```python
from build123d import *

# Parameters (mm, degrees)
F1_DEPTH = 6.3
F3_DEPTH = 4
F4_R     = 2.35
F4_R_2   = 1
F5_DEPTH = 3
F7_DEPTH = 2.5


with BuildPart() as f1:
    # F0 (on Top) → F1 (new body, symmetric)
    with BuildSketch(Plane.XY):
        Polygon((7.7, 11.4), (-8, 11.4), (-8, -11.4), (7.7, -11.4), (7.7, -16.25), (10.2, -16.25), (10.2, -11.4), (15, -11.4), (15, 11.4), (10.2, 11.4), (10.2, 16.25), (7.7, 16.25), align=None)
    extrude(amount=F1_DEPTH, both=True)

    # F2 (on face) → F3 (join)
    with BuildSketch(Plane.YZ.offset(15)):
        with BuildLine():
            ThreePointArc((5.1, 6.3), (1.0729415714, 4.844873622), (-1.0938378269, 1.1516826707))
            ThreePointArc((-1.0938378269, 1.1516826707), (-1.2, 0), (-1.0938378269, -1.1516826707))
            ThreePointArc((-1.0938378269, -1.1516826707), (1.072941559, -4.8448736116), (5.0999999676, -6.3))
            ThreePointArc((5.0999999676, -6.3), (9.55477271, -4.4547727329), (11.4, 0))
            ThreePointArc((11.4, 0), (9.5547727215, 4.4547727215), (5.1, 6.3))
        make_face()
        with BuildLine():
            ThreePointArc((-1.0938378269, -1.1516826707), (-1.2, 0), (-1.0938378269, 1.1516826707))
            ThreePointArc((-1.0938378269, 1.1516826707), (-2.8, 0), (-1.0938378269, -1.1516826707))
        make_face()
    extrude(amount=F3_DEPTH)

    # F4 (on face) → F5 (join)
    with BuildSketch(Plane.YZ.offset(19)):
        with Locations((5.1, 0)):
            Circle(F4_R)
        with Locations((5.1, 0)):
            Circle(F4_R_2, mode=Mode.SUBTRACT)
    extrude(amount=F5_DEPTH)

    # F6 (on face) → F7 (cut, through all)
    with BuildSketch(Plane.YZ.offset(10.2)):
        with BuildLine():
            ThreePointArc((14.6160254038, -0.5), (14.7159258263, -0.2588190451), (14.75, 0))
            ThreePointArc((14.75, 0), (14.7159258263, 0.2588190451), (14.6160254038, 0.5))
            ThreePointArc((14.6160254038, 0.5), (12.75, 0), (14.6160254038, -0.5))
        make_face()
        with BuildLine():
            ThreePointArc((14.6160254038, 0.5), (14.7159258263, 0.2588190451), (14.75, 0))
            ThreePointArc((14.75, 0), (14.7159258263, -0.2588190451), (14.6160254038, -0.5))
            Line((14.6160254038, -0.5), (16.25, -0.5))
            Line((16.25, -0.5), (16.25, 0.5))
            Line((16.25, 0.5), (14.6160254038, 0.5))
        make_face()
        with BuildLine():
            ThreePointArc((-14.6160254038, -0.5), (-13.4911809549, -0.9659258263), (-12.75, 0))
            ThreePointArc((-12.75, 0), (-13.4911809549, 0.9659258263), (-14.6160254038, 0.5))
            ThreePointArc((-14.6160254038, 0.5), (-14.75, 0), (-14.6160254038, -0.5))
        make_face()
        with BuildLine():
            ThreePointArc((-14.6160254038, -0.5), (-14.75, 0), (-14.6160254038, 0.5))
            Line((-14.6160254038, 0.5), (-16.25, 0.5))
            Line((-16.25, 0.5), (-16.25, -0.5))
            Line((-16.25, -0.5), (-14.6160254038, -0.5))
        make_face()
    extrude(amount=-F7_DEPTH, mode=Mode.SUBTRACT)


solid = f1.part
```
Can you work these out from the model? Positions are in its coordinate system, mm. A direction names the side the tool comes from. Round coordinates to 2 decimals unless told otherwise and drop trailing zeros. Order: outer loops, then holes, each group sorted by start corner. A loop starts at its lowest first (then second) coordinate and runs counter-clockwise, first axis right, second up. Notation, with made-up numbers: (-40, 49) -> (16, 49) arc R20 ccw to (16, 54) -> close; hole circle Ø6 at (-7, -36.5). An arc over 180 degrees is marked (long way). Return JSON: item names as keys, results as strings. Group by question number.
1. I need wall thicknesses on line 1 (Z direction, x = 20.4, y = 5.1); line 2 (X direction, y = 14, z = -1.25); line 3 (X direction, y = -6.5, z = -0.5). Which ranges of each line are inside material? Lowest first, please. Write a range as [from, to].
2. Which directions (+Z, -Z, +X, -X, +Y, -Y) give clear straight access to the entire face, cutting with the end or side of a thin tool? Please do faces 1 (the face through (7.7, 13.9, 1.5)), 2 (the face through (20.479, 4.591, -2.294)), 3 (the face through (15, 10, 5)), 4 (the face through (10.2, -13.9, 1.5)), 5 (the face through (9, 15, -0.5)).
3. If we section it at A-A, the plane y = 13.75: Write out the boundary of the cut face in (x, z), then the cut area to 3 significant figures.
4. We'd pull the mould along Z, two halves only. Please class faces 6 (the face through (19, 2.6, 0.1)), 7 (the face through (9, -15, 0.5)), 8 (the face through (3, 0, -6.3)): released by +Z, released by -Z, zero draft, split by the parting line, or undercut.
5. If we section it at B-B, the plane z = -3.75: Write out the boundary of the cut face in (x, y).
6. Will these pins go through, and if not, where does the flat tip stop? pin 1 (5.5 mm diameter, centred on y = -15, z = 0, fed in from +X); pin 2 (2 mm diameter, centred on y = -9.5, z = 2, fed in from +X); pin 3 (1.6 mm diameter, centred on y = 5.1, z = 0, fed in from +X).
7. If we section it at D-D, the plane y = -14: Write out the boundary of the cut face in (x, z), then the cut area to 3 significant figures.
Output values:
{
 "1": {"line 1": "[-2.35, -1], [1, 2.35]", "line 2": "[7.7, 10.2]", "line 3": "[-8, 15]"},
 "2": {"face 1": "+Z, -Z, -X, +Y", "face 2": "+X", "face 3": "+Z, +X, +Y", "face 4": "+Z, -Z, +X, -Y", "face 5": "+X, -X, +Y"},
 "3": {"outline": "(7.7, -6.3) -> (10.2, -6.3) -> (10.2, -1) -> (7.7, -1) -> close; (7.7, 1) -> (10.2, 1) -> (10.2, 6.3) -> (7.7, 6.3) -> close", "area": "26.5 mm²"},
 "4": {"face 6": "zero draft", "face 7": "undercut", "face 8": "released by -Z"},
 "5": {"outline": "(-8, -11.4) -> (7.7, -11.4) -> (7.7, -16.25) -> (10.2, -16.25) -> (10.2, -11.4) -> (15, -11.4) -> (15, 0.04) -> (19, 0.04) -> (19, 10.16) -> (15, 10.16) -> (15, 11.4) -> (10.2, 11.4) -> (10.2, 16.25) -> (7.7, 16.25) -> (7.7, 11.4) -> (-8, 11.4) -> close"},
 "6": {"pin 1": "x = 10.2", "pin 2": "x = 15", "pin 3": "x = 19"},
 "7": {"outline": "(7.7, -6.3) -> (10.2, -6.3) -> (10.2, -0.97) -> (7.7, -0.97) -> close; (7.7, 0.97) -> (10.2, 0.97) -> (10.2, 6.3) -> (7.7, 6.3) -> close", "area": "26.7 mm²"}
}
